Can you work these out from the drawing? Everything is in mm from the part's minimum corner. Round coordinates to 2 decimals unless told otherwise and drop trailing zeros. Loops run counter-clockwise (first coordinate to the right, second up) from the corner with the lowest first, then second, coordinate; pieces in that order, holes last. Notation, with made-up numbers: (34, 44) - (83, 44) arc R13 cw to (83, 62) - close; hole circle Ø1 at (-39.5, -27). An arc over 180 degrees is marked (long way). Answer as a JSON object with one key per item and string values. Group by question number.
1) I want a section at B-B, the plane z = 44. Please give me the cut outline in (x, y).
2) I want a section at A-A, the plane y = 1.15. Please give me the cut outline in (x, z).
3) Will this pin go through, and if not, where does the flat tip stop? P1, Ø0.8, axis at y = 1, z = 24.5, coming from the -X side.
4) If I drill on line 1 along X through (y, z) = (1.45, 52); line 2 along Z through (x, y) = (71, 2.25), over which ranges is the centre line in solid material (lowest first)? Write a range as [from, to].
5) I want a section at C-C, the plane x = 96. Please give me the cut outline in (y, z), then the cut area to 4 significant figures.
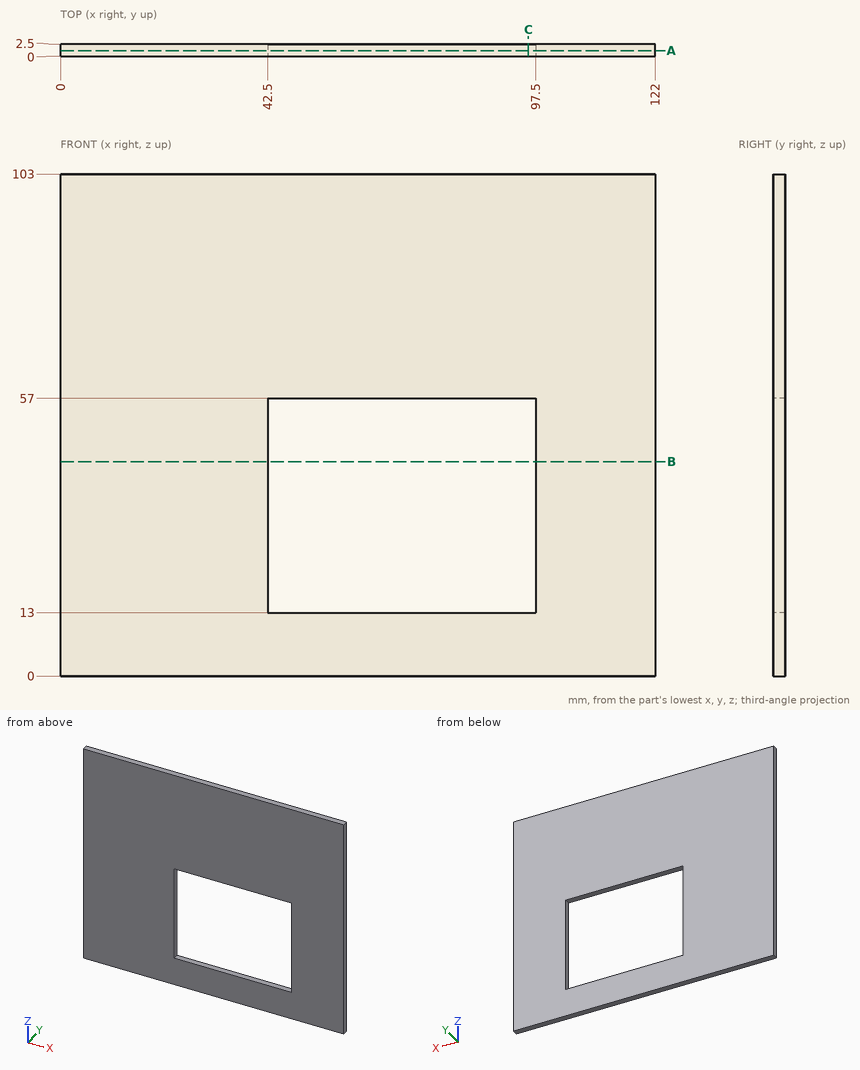
Outcome:
{
 "1": {"outline": "(0, 0) - (42.5, 0) - (42.5, 2.5) - (0, 2.5) - close; (97.5, 0) - (122, 0) - (122, 2.5) - (97.5, 2.5) - close"},
 "2": {"outline": "(0, 0) - (122, 0) - (122, 103) - (0, 103) - close; hole (42.5, 13) - (97.5, 13) - (97.5, 57) - (42.5, 57) - close"},
 "3": {"P1": "x = 0"},
 "4": {"line 1": "[0, 42.5], [97.5, 122]", "line 2": "[0, 13], [57, 103]"},
 "5": {"outline": "(0, 0) - (2.5, 0) - (2.5, 13) - (0, 13) - close; (0, 57) - (2.5, 57) - (2.5, 103) - (0, 103) - close", "area": "147.5 mm^2"}
}
